Check sheet for the modelled part. Datum: model origin and axes. Units: mm. A direction names the side the tool comes from. Coordinates: 2 decimals unless noted, no trailing zeros. Loops run counter-clockwise (first coordinate to the right, second up) from the corner with the lowest first, then second, coordinate; pieces in that order, holes last. Notation, with made-up numbers: (-37.5, 74.25) -> (16.5, 74.25) arc R16 cw to (16.5, 102.25) -> close; hole circle Ø7 at (49.5, 52). An arc over 180 degrees is marked (long way). Use one line per item in the form item = value.
from build123d import *

# Parameters (mm, degrees)
ESQUISSE1_R        = 4.502635458
BOSS_EXTRU_1_DEPTH = 10
D_GAGEMENT_M21_D   = 2.4
CONG_1_R           = 10
D_GAGEMENT_M61_D   = 6.6


with BuildPart() as part:
    # Esquisse1 → Boss.-Extru.1 (new body)
    with BuildSketch(Plane.XY):
        with BuildLine():
            Line((-7, 38), (-7, -38))
            ThreePointArc((-7, -38), (0, -57.485281374), (7, -38))
            Line((7, -38), (7, 38))
            ThreePointArc((7, 38), (0, 57.485281374), (-7, 38))
        make_face()
        with Locations((0, 46.485281374)):
            Circle(ESQUISSE1_R, mode=Mode.SUBTRACT)
    extrude(amount=BOSS_EXTRU_1_DEPTH)

    # Dégagement M21 (through all)
    with Locations(Plane.XY.offset(10)):
        with Locations((-8, 46.485281374), (0, 54.485281374), (8, 46.485281374), (0, 38.485281374)):
            Hole(D_GAGEMENT_M21_D / 2)

    # Congé1
    cong_1_edges = [part.edges().sort_by_distance(p)[0] for p in [
        (7, 38, 5),
        (7, -38, 5),
        (-7, -38, 5),
        (-7, 38, 5),
    ]]
    fillet(cong_1_edges, radius=CONG_1_R)

    # Dégagement M61 (through all)
    with Locations(Plane.XY.offset(10)):
        with Locations((0, -46.485281374)):
            Hole(D_GAGEMENT_M61_D / 2)


solid = part.part
(1) Section check D-D, the plane x = -5.5. Record the boundary of the cut face in (y, z).
Established:
outline = (-56.01, 0) -> (56.01, 0) -> (56.01, 10) -> (-56.01, 10) -> close
(2) Section check A-A, the plane x = 0. Record the boundary of the cut face in (y, z).
Established:
outline = (-57.49, 0) -> (-49.79, 0) -> (-49.79, 10) -> (-57.49, 10) -> close; (-43.19, 0) -> (37.29, 0) -> (37.29, 10) -> (-43.19, 10) -> close; (39.69, 0) -> (41.98, 0) -> (41.98, 10) -> (39.69, 10) -> close; (50.99, 0) -> (53.29, 0) -> (53.29, 10) -> (50.99, 10) -> close; (55.69, 0) -> (57.49, 0) -> (57.49, 10) -> (55.69, 10) -> close
(3) Section check C-C, the plane y = 2.5. Record the boundary of the cut face in (x, z).
Established:
outline = (-7, 0) -> (7, 0) -> (7, 10) -> (-7, 10) -> close
(4) Mould release check, pull along X, two halves, no side actions. Record for faces 1 (the cylindrical face through (-0.34, -57.48, 4.93)), 2 (the cylindrical face through (8.88, 47.3, 4.93)), 3 (the flat face through (-7, 0, 5)), 4 (the cylindrical face through (0.715, -49.707, 4.93)): +X half, -X half, draft (parallel to the pull), parting line (faces both ways), or undercut.
Established:
face_1 = parting line
face_2 = undercut
face_3 = -X half
face_4 = undercut
(5) Go/stop test with flat-tipped pins: P1, Ø5, axis at y = -8, z = 2.5, coming from the -X side; P2, Ø3, axis at x = 2.5, z = 7.5, coming from the +Y side; P3, Ø3, axis at y = 0, z = 3.5, coming from the +X side. Record where each tip stops, or that it passes through.
Established:
P1 = -7
P2 = 57.44
P3 = 7
(6) Tool access check on faces 5 (the flat face through (7, 0, 5)), 6 (the cylindrical face through (-6.8, 46.5, 4.9)), 7 (the cylindrical face through (-7.475, -37.201, 5.07)). Record the directions out of +Z, -Z, +X, -X, +Y, -Y that give a thin tool (end or side, any length) a straight path to the whole face; none if there is none.
Established:
face_5 = +Z, -Z, +X
face_6 = +Z, -Z
face_7 = +Z, -Z, -X
(7) Scan lines: line 1 along Y through (x, z) = (0, 5.5); line 2 along Y through (x, z) = (9, 5); line 3 along Y through (x, z) = (3, 7). Record each from-to range of solid material in increasing order.
Established:
line_1 = -57.49 to -49.79, -43.19 to 37.29, 39.69 to 41.98, 50.99 to 53.29, 55.69 to 57.49
line_2 = -52.81 to -40.16, 40.16 to 45.82, 47.15 to 52.81
line_3 = -57.07 to -47.86, -45.11 to 43.13, 49.84 to 57.07
(8) Section check B-B, the plane z = 3. Record the boundary of the cut face in (x, y).
Established:
outline = (-8.9, -40.03) arc R11 ccw (long way) to (8.9, -40.03) arc R10 cw to (7, -34.16) -> (7, 34.16) arc R10 cw to (8.9, 40.03) arc R11 ccw (long way) to (-8.9, 40.03) arc R10 cw to (-7, 34.16) -> (-7, -34.16) arc R10 cw to start; hole circle Ø2.4 at (-8, 46.49); hole circle Ø9.01 at (0, 46.49); hole circle Ø6.6 at (0, -46.49); hole circle Ø2.4 at (0, 38.49); hole circle Ø2.4 at (0, 54.49); hole circle Ø2.4 at (8, 46.49)
